Design review of the part built by this model. Coordinates are the model's own, in mm. A direction names the side the tool comes from. Give positions to 0.01 mm unless a question says otherwise; leave off trailing zeros. Write each loop counter-clockwise with the first axis right and the second up, starting at its lowest first coordinate (ties: lowest second). Pieces come first, ordered by that corner, then holes. Notation, with made-up numbers: (-34, 43) -> (-19, 43) arc R9 ccw to (-19, 59) -> close; hole circle Ø11 at (75.5, 17). An arc over 180 degrees is marked (long way). Use CSV: the item, a comma, the result in double quotes.
```python
from build123d import *
from OCP.BRepFilletAPI import BRepFilletAPI_MakeChamfer

# Parameters (mm, degrees)
ESQUISSE1_W             = 18
ESQUISSE1_H             = 14
BOSS_EXTRU_1_DEPTH      = 1.5
ESQUISSE4_W             = 1.5
ESQUISSE4_H             = 2.5
BOSS_EXTRU_4_DEPTH      = 1
ESQUISSE5_W             = 17.8
ESQUISSE5_H             = 1.8
BOSS_EXTRU_5_DEPTH      = 3
BOSS_EXTRU_6_DEPTH      = 10
BOSS_EXTRU_6_DEPTH_BACK = 6
ESQUISSE6_R             = 0.486228561
CHANFREIN2_SIZE         = 0.5
CHANFREIN2_SIZE2        = 0.288675135
ESQUISSE7_W             = 2.5
ESQUISSE7_H             = 9.31757076
ENL_V_MAT_EXTRU_1_DEPTH = 27.195610319
CHANFREIN3_SIZE         = 0.4
CHANFREIN3_SIZE2        = 0.230940108
ESQUISSE8_W             = 6
ESQUISSE8_H             = 6
BOSS_EXTRU_7_DEPTH      = 1.5


with BuildPart() as part:
    # Esquisse1 → Boss.-Extru.1 (new body)
    with BuildSketch(Plane.XY):
        with Locations((9, 7)):
            Rectangle(ESQUISSE1_W, ESQUISSE1_H)
    extrude(amount=BOSS_EXTRU_1_DEPTH)

    # Esquisse4 → Boss.-Extru.4 (add)
    with BuildSketch(Plane.XY.offset(1.5)):
        with Locations((0.75, 8.75)):
            Rectangle(ESQUISSE4_W, ESQUISSE4_H)
    extrude(amount=BOSS_EXTRU_4_DEPTH)

    # Esquisse5 → Boss.-Extru.5 (add)
    with BuildSketch(Plane(origin=(0, 0, 0), x_dir=(-1, 0, 0), z_dir=(0, 0, -1))):
        with Locations((-9, 13)):
            Rectangle(ESQUISSE5_W, ESQUISSE5_H)
    extrude(amount=BOSS_EXTRU_5_DEPTH)

    # Esquisse6 → Boss.-Extru.6 (add, two sides: drawn at the far end of the back side and taken through both)
    with BuildSketch(Plane(origin=(0, 0, -3), x_dir=(-1, 0, 0), z_dir=(0, 0, -1)).offset(-BOSS_EXTRU_6_DEPTH_BACK)):
        with Locations((-1.38, 13)):
            Circle(ESQUISSE6_R)
        with Locations((-3.92, 13)):
            Circle(ESQUISSE6_R)
        with Locations((-6.46, 13)):
            Circle(ESQUISSE6_R)
        with Locations((-9, 13)):
            Circle(ESQUISSE6_R)
        with Locations((-11.54, 13)):
            Circle(ESQUISSE6_R)
        with Locations((-14.08, 13)):
            Circle(ESQUISSE6_R)
        with Locations((-16.62, 13)):
            Circle(ESQUISSE6_R)
    extrude(amount=BOSS_EXTRU_6_DEPTH + BOSS_EXTRU_6_DEPTH_BACK)

    # Chanfrein2: one chamfer whose edges measure the first distance from different faces: ONE call of the kernel's chamfer builder (chamfer() names one face for all edges)
    chanfrein2_edges_1 = [part.edges().sort_by_distance(p)[0] for p in [
        (1.866228561, 13, -13),
    ]]
    chanfrein2_side_1 = [part.faces().sort_by_distance(p)[0] for p in [
        (1.866228561, 13, -8),
    ]]
    chanfrein2_edges_2 = [part.edges().sort_by_distance(p)[0] for p in [
        (4.406228561, 13, -13),
    ]]
    chanfrein2_side_2 = [part.faces().sort_by_distance(p)[0] for p in [
        (4.406228561, 13, -8),
    ]]
    chanfrein2_edges_3 = [part.edges().sort_by_distance(p)[0] for p in [
        (6.946228561, 13, -13),
    ]]
    chanfrein2_side_3 = [part.faces().sort_by_distance(p)[0] for p in [
        (6.946228561, 13, -8),
    ]]
    chanfrein2_edges_4 = [part.edges().sort_by_distance(p)[0] for p in [
        (9.486228561, 13, -13),
    ]]
    chanfrein2_side_4 = [part.faces().sort_by_distance(p)[0] for p in [
        (9.486228561, 13, -8),
    ]]
    chanfrein2_edges_5 = [part.edges().sort_by_distance(p)[0] for p in [
        (12.026228561, 13, -13),
    ]]
    chanfrein2_side_5 = [part.faces().sort_by_distance(p)[0] for p in [
        (12.026228561, 13, -8),
    ]]
    chanfrein2_edges_6 = [part.edges().sort_by_distance(p)[0] for p in [
        (14.566228561, 13, -13),
    ]]
    chanfrein2_side_6 = [part.faces().sort_by_distance(p)[0] for p in [
        (14.566228561, 13, -8),
    ]]
    chanfrein2_edges_7 = [part.edges().sort_by_distance(p)[0] for p in [
        (17.106228561, 13, -13),
    ]]
    chanfrein2_side_7 = [part.faces().sort_by_distance(p)[0] for p in [
        (17.106228561, 13, -8),
    ]]
    chanfrein2 = BRepFilletAPI_MakeChamfer(part.part.solid().wrapped)
    for e in chanfrein2_edges_1:
        chanfrein2.Add(CHANFREIN2_SIZE, CHANFREIN2_SIZE2, e.wrapped, chanfrein2_side_1[0].wrapped)  # the first distance lies on this face
    for e in chanfrein2_edges_2:
        chanfrein2.Add(CHANFREIN2_SIZE, CHANFREIN2_SIZE2, e.wrapped, chanfrein2_side_2[0].wrapped)  # the first distance lies on this face
    for e in chanfrein2_edges_3:
        chanfrein2.Add(CHANFREIN2_SIZE, CHANFREIN2_SIZE2, e.wrapped, chanfrein2_side_3[0].wrapped)  # the first distance lies on this face
    for e in chanfrein2_edges_4:
        chanfrein2.Add(CHANFREIN2_SIZE, CHANFREIN2_SIZE2, e.wrapped, chanfrein2_side_4[0].wrapped)  # the first distance lies on this face
    for e in chanfrein2_edges_5:
        chanfrein2.Add(CHANFREIN2_SIZE, CHANFREIN2_SIZE2, e.wrapped, chanfrein2_side_5[0].wrapped)  # the first distance lies on this face
    for e in chanfrein2_edges_6:
        chanfrein2.Add(CHANFREIN2_SIZE, CHANFREIN2_SIZE2, e.wrapped, chanfrein2_side_6[0].wrapped)  # the first distance lies on this face
    for e in chanfrein2_edges_7:
        chanfrein2.Add(CHANFREIN2_SIZE, CHANFREIN2_SIZE2, e.wrapped, chanfrein2_side_7[0].wrapped)  # the first distance lies on this face
    add(Compound.cast(chanfrein2.Shape()), mode=Mode.REPLACE)

    # Esquisse7 → Enlèv. mat.-Extru.1 (cut, through all)
    with BuildSketch(Plane(origin=(0, 13.9, 0), x_dir=(1, 0, 0), z_dir=(0, 1, 0))):
        with Locations((1.25, 8.65878538)):
            Rectangle(ESQUISSE7_W, ESQUISSE7_H)
    extrude(amount=-ENL_V_MAT_EXTRU_1_DEPTH, mode=Mode.SUBTRACT)

    # Chanfrein3: one chamfer whose edges measure the first distance from different faces: ONE call of the kernel's chamfer builder (chamfer() names one face for all edges)
    chanfrein3_edges_1 = [part.edges().sort_by_distance(p)[0] for p in [
        (1.866228561, 13, 3),
    ]]
    chanfrein3_side_1 = [part.faces().sort_by_distance(p)[0] for p in [
        (1.38, 13, 3),
    ]]
    chanfrein3_edges_2 = [part.edges().sort_by_distance(p)[0] for p in [
        (4.406228561, 13, 3),
    ]]
    chanfrein3_side_2 = [part.faces().sort_by_distance(p)[0] for p in [
        (3.92, 13, 3),
    ]]
    chanfrein3_edges_3 = [part.edges().sort_by_distance(p)[0] for p in [
        (6.946228561, 13, 3),
    ]]
    chanfrein3_side_3 = [part.faces().sort_by_distance(p)[0] for p in [
        (6.46, 13, 3),
    ]]
    chanfrein3_edges_4 = [part.edges().sort_by_distance(p)[0] for p in [
        (9.486228561, 13, 3),
    ]]
    chanfrein3_side_4 = [part.faces().sort_by_distance(p)[0] for p in [
        (9, 13, 3),
    ]]
    chanfrein3_edges_5 = [part.edges().sort_by_distance(p)[0] for p in [
        (12.026228561, 13, 3),
    ]]
    chanfrein3_side_5 = [part.faces().sort_by_distance(p)[0] for p in [
        (11.54, 13, 3),
    ]]
    chanfrein3_edges_6 = [part.edges().sort_by_distance(p)[0] for p in [
        (14.566228561, 13, 3),
    ]]
    chanfrein3_side_6 = [part.faces().sort_by_distance(p)[0] for p in [
        (14.08, 13, 3),
    ]]
    chanfrein3_edges_7 = [part.edges().sort_by_distance(p)[0] for p in [
        (17.106228561, 13, 3),
    ]]
    chanfrein3_side_7 = [part.faces().sort_by_distance(p)[0] for p in [
        (16.62, 13, 3),
    ]]
    chanfrein3 = BRepFilletAPI_MakeChamfer(part.part.solid().wrapped)
    for e in chanfrein3_edges_1:
        chanfrein3.Add(CHANFREIN3_SIZE, CHANFREIN3_SIZE2, e.wrapped, chanfrein3_side_1[0].wrapped)  # the first distance lies on this face
    for e in chanfrein3_edges_2:
        chanfrein3.Add(CHANFREIN3_SIZE, CHANFREIN3_SIZE2, e.wrapped, chanfrein3_side_2[0].wrapped)  # the first distance lies on this face
    for e in chanfrein3_edges_3:
        chanfrein3.Add(CHANFREIN3_SIZE, CHANFREIN3_SIZE2, e.wrapped, chanfrein3_side_3[0].wrapped)  # the first distance lies on this face
    for e in chanfrein3_edges_4:
        chanfrein3.Add(CHANFREIN3_SIZE, CHANFREIN3_SIZE2, e.wrapped, chanfrein3_side_4[0].wrapped)  # the first distance lies on this face
    for e in chanfrein3_edges_5:
        chanfrein3.Add(CHANFREIN3_SIZE, CHANFREIN3_SIZE2, e.wrapped, chanfrein3_side_5[0].wrapped)  # the first distance lies on this face
    for e in chanfrein3_edges_6:
        chanfrein3.Add(CHANFREIN3_SIZE, CHANFREIN3_SIZE2, e.wrapped, chanfrein3_side_6[0].wrapped)  # the first distance lies on this face
    for e in chanfrein3_edges_7:
        chanfrein3.Add(CHANFREIN3_SIZE, CHANFREIN3_SIZE2, e.wrapped, chanfrein3_side_7[0].wrapped)  # the first distance lies on this face
    add(Compound.cast(chanfrein3.Shape()), mode=Mode.REPLACE)

    # Esquisse8 → Boss.-Extru.7 (add)
    with BuildSketch(Plane.XY.offset(1.5)):
        with Locations((13, 5)):
            Rectangle(ESQUISSE8_W, ESQUISSE8_H)
    extrude(amount=BOSS_EXTRU_7_DEPTH)


solid = part.part
```
(1) Mouldability with a two-part tool opening along X and no side actions: class faces 4 (the face through (13, 2, 2)), 5 (the face through (16.171, 12.814, -7.683)), 6 (the face through (3.696, 12.569, -7.683)) as +X half, -X half, draft (parallel to the pull), parting line (faces both ways), or undercut.
Established:
face 4,"draft"
face 5,"undercut"
face 6,"undercut"
(2) Take a section at C-C (z = -9.75). Write out the cut boundary in (x, y).
Established:
outline,"circle Ø0.97 at (3.92, 13); circle Ø0.97 at (6.46, 13); circle Ø0.97 at (9, 13); circle Ø0.97 at (11.54, 13); circle Ø0.97 at (14.08, 13); circle Ø0.97 at (16.62, 13)"
(3) Take a section at A-A (z = -3.5). Write out the cut boundary in (x, y), then the cut area to 3 significant figures.
Established:
outline,"circle Ø0.97 at (1.38, 13); circle Ø0.97 at (3.92, 13); circle Ø0.97 at (6.46, 13); circle Ø0.97 at (9, 13); circle Ø0.97 at (11.54, 13); circle Ø0.97 at (14.08, 13); circle Ø0.97 at (16.62, 13)"
area,"5.20 mm2"
(4) Clearance check with flat-ended pins moving along their axes: pin 1 (0.5 mm diameter, centred on x = 1.5, y = 13, fed in from -Z); pin 2 (0.8 mm diameter, centred on x = 0.5, z = 2, fed in from -Y); pin 3 (1.2 mm diameter, centred on x = 1, y = 8.5, fed in from +Z). State where each tip first meets the part, or that it passes through.
Established:
pin 1,"stops at z = -4"
pin 2,"stops at y = 7.5"
pin 3,"stops at z = 2.5"
(5) Tool access review of faces 1 (the face through (8.536, 13.146, 2.143)), 2 (the face through (1, 9, 2.5)), 3 (the face through (1.4, 13, -4)): name each direction out of +Z, -Z, +X, -X, +Y, -Y from which nothing blocks a thin tool from reaching the whole face with its end or side.
Established:
face 1,"+Z"
face 2,"+Z, -X, -Y"
face 3,"-Z, -X, +Y, -Y"
(6) Take a section at D-D (y = 9). Write out the cut boundary in (x, z).
Established:
outline,"(0, 0) -> (18, 0) -> (18, 1.5) -> (1.5, 1.5) -> (1.5, 2.5) -> (0, 2.5) -> close"
(7) For line 1 along X through (y, z) = (13, -1.75); line 2 along Y through (x, z) = (6, -2.75); line 3 along Y through (x, z) = (6.5, -4.25), list the stretches that pass through material, from the lowest coordinate up. Write a range as [from, to].
Established:
line 1,"x = [0.1, 17.9]"
line 2,"y = [12.1, 13.9]"
line 3,"y = [12.52, 13.48]"
(8) Take a section at B-B (x = 7.5). Write out the cut boundary in (y, z).
Established:
outline,"(0, 0) -> (12.1, 0) -> (12.1, -3) -> (13.9, -3) -> (13.9, 0) -> (14, 0) -> (14, 1.5) -> (0, 1.5) -> close"
